The model under review builds one solid part; all positions refer to its coordinate system, in mm. Face numbers are marked on the shaded views. Round coordinates to 2 decimals unless told otherwise and drop trailing zeros. Order: outer loops, then holes, each group sorted by start corner. A loop starts at its lowest first (then second) coordinate and runs counter-clockwise, first axis right, second up. Notation, with made-up numbers: (10, 3) -> (55, 3) arc R25 cw to (55, 39) -> close; hole circle Ø5 at (71, -19.5). An arc over 180 degrees is marked (long way). Use a Markdown table: item, result. Add a question column.
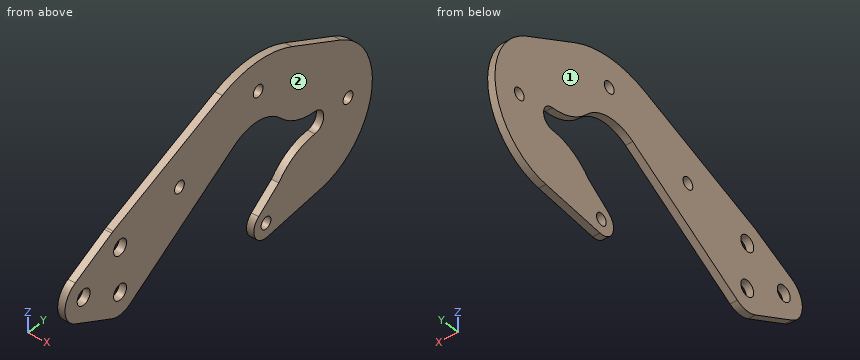
```python
from build123d import *

# Parameters (mm, degrees)
SKETCH1_R              = 3.3782
BOSS_EXTRUDE1_DEPTH    = 3.175
F_10_CLEARANCE_HOLE1_D = 5.1054


with BuildPart() as part:
    # Sketch1 → Boss-Extrude1 (new body)
    with BuildSketch(Plane(origin=(0, 0, 0), x_dir=(0, 0, -1), z_dir=(1, 0, 0))):
        with BuildLine():
            Line((-16.180222385, 59.795006038), (17.787700231, 5.13475025))
            ThreePointArc((17.787700231, 5.13475025), (19.242822935, 0.449213357), (18.226166599, -4.3505833))
            Line((18.226166599, -4.3505833), (8.701166599, -23.4005833))
            ThreePointArc((8.701166599, -23.4005833), (0, -28.7782), (-8.701166599, -23.4005833))
            Line((-8.701166599, -23.4005833), (-18.226166599, -4.3505833))
            ThreePointArc((-18.226166599, -4.3505833), (-18.401518048, -3.980615854), (-18.561147274, -3.603597881))
            Line((-18.561147274, -3.603597881), (-41.287879188, 53.384474435))
            ThreePointArc((-41.287879188, 53.384474435), (-44.407665238, 71.789527798), (-39.695119269, 89.8525))
            Line((-39.695119269, 89.8525), (-26.935973789, 115.173125))
            ThreePointArc((-26.935973789, 115.173125), (5.234726153, 131.304781574), (29.953116968, 105.147843028))
            Line((29.953116968, 105.147843028), (33.293419362, 76.946914322))
            ThreePointArc((33.293419362, 76.946914322), (29.346967441, 70.304627798), (21.9075, 72.39))
            Line((21.9075, 72.39), (14.051055193, 82.865259743))
            ThreePointArc((14.051055193, 82.865259743), (7.358887034, 91.297415515), (4.760318612, 101.744128289))
            ThreePointArc((4.760318612, 101.744128289), (0, 106.3625), (-4.760318612, 101.744128289))
            ThreePointArc((-4.760318612, 101.744128289), (-7.038090513, 91.974290609), (-12.920864804, 83.848348214))
            ThreePointArc((-12.920864804, 83.848348214), (-18.877476959, 72.407999932), (-16.180222385, 59.795006038))
        make_face()
        with Locations((9.525, 0)):
            Circle(SKETCH1_R, mode=Mode.SUBTRACT)
        with Locations((-9.525, 0)):
            Circle(SKETCH1_R, mode=Mode.SUBTRACT)
        with Locations((0, -19.05)):
            Circle(SKETCH1_R, mode=Mode.SUBTRACT)
    extrude(amount=BOSS_EXTRUDE1_DEPTH)

    # #10 Clearance Hole1 (through all)
    with Locations(Plane(origin=(3.175, 0, 0), x_dir=(0, 0, -1), z_dir=(1, 0, 0))):
        with Locations((-16.086295304, 31.002116448), (-31.642571099, 72.098763865), (0, 119.0625), (26.9875, 76.2)):
            Hole(F_10_CLEARANCE_HOLE1_D / 2)


solid = part.part
```
Q1. For pin 1 (4 mm diameter, centred on y = -19.05, z = 0, fed in from -X), flat-tipped, find the tip position at first contact; note if it passes through.
Q2. Add section D-D, the plane z = 0. Give the boundary of the cut face in (x, y) (1 decimal), then the cut area to 3 significant figures.
Q3. Add section A-A, the plane y = 81. Give the boundary of the cut face in (x, z) (3 decimals).
Q4. Draft analysis for pull direction X (two halves, no side actions). For the marked faces 1 and 2, state which applies: released by +X, released by -X, zero draft, split by the parting line, or undercut.
Q5. Add section B-B, the plane x = 0.95. Give the number of separate pieces and of enclosed holes in the cut face, then the cut area to 3 significant figures.
Q6. Add section C-C, the plane y = 0. Give the boundary of the cut face in (x, z) (3 decimals).
Q7. To check wall thickness, follow line 1 along Y through (x, z) = (1.3, 15.5); line 2 along Y through (x, z) = (0.6, 2); line 3 along Y through (x, z) = (1.5, 0). State the ranges of each line that lie inside material, in increasing order.
Return value:
| question | item | result |
|---|---|---|
| 1 | pin 1 | through |
| 2 | outline | (0, -28.8) -> (3.2, -28.8) -> (3.2, -22.4) -> (0, -22.4) -> close; (0, -15.7) -> (3.2, -15.7) -> (3.2, 33.8) -> (0, 33.8) -> close; (0, 106.4) -> (3.2, 106.4) -> (3.2, 116.5) -> (0, 116.5) -> close; (0, 121.6) -> (3.2, 121.6) -> (3.2, 131.8) -> (0, 131.8) -> close |
| 2 | area | 242 mm² |
| 3 | outline | (0, -32.813) -> (3.175, -32.813) -> (3.175, -15.45) -> (0, -15.45) -> close; (0, 15.446) -> (3.175, 15.446) -> (3.175, 43.029) -> (0, 43.029) -> close |
| 4 | face 1 | released by -X |
| 4 | face 2 | released by +X |
| 5 | separate pieces | 1 |
| 5 | enclosed holes | 7 |
| 5 | area | 5,810 mm² |
| 6 | outline | (0, -19.253) -> (3.175, -19.253) -> (3.175, -12.903) -> (0, -12.903) -> close; (0, -6.147) -> (3.175, -6.147) -> (3.175, 6.147) -> (0, 6.147) -> close; (0, 12.903) -> (3.175, 12.903) -> (3.175, 19.998) -> (0, 19.998) -> close |
| 7 | line 1 | -9.8 to 28.52, 33.49 to 58.7, 80.92 to 127.48 |
| 7 | line 2 | -28.57 to -21.77, -16.33 to 36.98, 105.92 to 117.48, 120.65 to 131.7 |
| 7 | line 3 | -28.78 to -22.43, -15.67 to 33.76, 106.36 to 116.51, 121.62 to 131.76 |
